Geometry: final body of the model. Coordinates: model frame, mm. A direction names the side the tool comes from. Give positions to 0.01 mm unless a question says otherwise; leave off trailing zeros. Order: outer loops, then holes, each group sorted by start corner. A loop starts at its lowest first (then second) coordinate and runs counter-clockwise, first axis right, second up. Notation, with made-up numbers: (74, -12.5) - (93, -12.5) arc R29 ccw to (93, 7.5) - close; hole circle Ø4 at (78, 21). An arc over 180 degrees is marked (long way). Use one line per item in the form item = value.
from build123d import *

# Parameters (mm, degrees)
F1_DEPTH = 15.24
F2_DEPTH = 12.192
F3_DEPTH = 9.144
F4_DEPTH = 6.096


with BuildPart() as f1:
    # F0 (on Top) → F1 (new body)
    with BuildSketch(Plane.XY):
        Polygon((-19.076721, 37.150636), (-54.891605, 37.150636), (-76.409116, -37.150636), (-40.594233, -37.150636), align=None)
        Polygon((-61.239227, -25.750598), (-46.324576, 25.750598), (-34.24661, 25.750598), (-49.161262, -25.750598), align=None, mode=Mode.SUBTRACT)
    extrude(amount=F1_DEPTH)

    # F0 (on Top) → F2 (join)
    with BuildSketch(Plane.XY):
        Polygon((-6.884721, 37.150636), (-19.076721, 37.150636), (-40.594233, -37.150636), (-24.240132, -37.150636), (-17.038353, -28.016673), (-14.754863, -37.150636), (-5.972206, -37.150636), (15.545306, 37.150636), (5.307279, 37.150636), (-9.230042, -13.047613), (-12.835056, -3.14023), (-21.369147, -12.864963), align=None)
    extrude(amount=F2_DEPTH)

    # F0 (on Top) → F3 (join)
    with BuildSketch(Plane.XY):
        Polygon((43.298501, 37.150636), (15.545306, 37.150636), (-5.972206, -37.150636), (21.78099, -37.150636), (25.299825, -24.999883), (11.423228, -24.999883), (17.365993, -4.479155), (26.523624, -4.479155), (29.117934, 4.479155), (26.523624, 4.479155), (19.960303, 4.479155), (25.932101, 25.100136), (39.808699, 25.100136), align=None)
    extrude(amount=F3_DEPTH)

    # F0 (on Top) → F4 (join)
    with BuildSketch(Plane.XY):
        Polygon((57.90846, 37.150636), (43.298501, 37.150636), (39.808699, 25.100136), (25.299825, -24.999883), (21.78099, -37.150636), (35.253152, -37.150636), (46.813049, 2.766387), (46.813049, -7.282906), (46.813049, -37.150636), (49.582697, -37.150636), (63.912243, -37.150636), (85.429754, 37.150636), (73.237754, 37.150636), (57.90846, -15.782347), align=None)
    extrude(amount=F4_DEPTH)


solid = f1.part
(1) Cut plane B-B on z = 2.5. Give the number of separate pieces and of enclosed holes in the cut face, plus the area to 3 significant figures.
Computed values:
separate_pieces = 1
enclosed_holes = 2
area = 7,960 mm²
(2) Contact query for flat-ended pins moving along their axis: pin 1 Ø5 at (y, z) = (-10, 3) entering from +X; pin 2 Ø5 at (y, z) = (-11, 3) entering from -X; pin 3 Ø4 at (y, z) = (27.5, 2) entering from +X. Output: stop coordinate, or through.
Computed values:
pin_1 = 72.5
pin_2 = -69.56
pin_3 = 83.21
(3) Reachability of faces 4 (the face through (79, 37.151, 3)), 5 (the face through (65.68, 11.05, 3.01)), 6 (the face through (14.353, -14.883, 4.508)), 7 (the face through (-20.69, -32.65, 6.01)), 8 (the face through (18, 1, 9.144)) from +Z, -Z, +X, -X, +Y, -Y: full face, straight path, thin tool, end or side. Return the list, or none.
Computed values:
face_4 = +Z, -Z, +X, -X, +Y
face_5 = +Z, -Z, +Y
face_6 = +Z, -Z
face_7 = +Z, -Z, -Y
face_8 = +Z, +X, -Y
(4) Ray query, line 1 along X through (y, z) = (-20.5, 5.25); line 2 along X through (y, z) = (-12, 11.5); line 3 along X through (y, z) = (14, 9). Return the intervals inside material, ascending.
Computed values:
line_1 = -71.59 to -59.72, -47.64 to 12.73, 26.6 to 40.08, 46.81 to 68.73
line_2 = -69.13 to -57.26, -45.18 to -21.12, -20.61 to -9.61, -8.93 to 1.31
line_3 = -61.6 to -49.73, -37.65 to -13.59, -1.4 to 22.72
(5) Cut plane A-A on z = 10.75. Output: boundary loops of the cut face in (x, y), plus the area to 3 significant figures.
Computed values:
outline = (-76.41, -37.15) - (-24.24, -37.15) - (-17.04, -28.02) - (-14.75, -37.15) - (-5.97, -37.15) - (15.55, 37.15) - (5.31, 37.15) - (-9.23, -13.05) - (-12.84, -3.14) - (-21.37, -12.86) - (-6.88, 37.15) - (-54.89, 37.15) - close; hole (-61.24, -25.75) - (-49.16, -25.75) - (-34.25, 25.75) - (-46.32, 25.75) - close
area = 4,020 mm²
(6) Pull-direction query (X, two-part tool) for faces 1 (the face through (18, -25, 5)), 2 (the face through (3, 1, 0)), 3 (the face through (-29.986, -0.52, 13.695)); classes: released by +X, released by -X, zero draft, split by the parting line, or undercut.
Computed values:
face_1 = undercut
face_2 = zero draft
face_3 = released by +X
(7) Cut plane D-D on y = -32. Output: boundary loops of the cut face in (x, z).
Computed values:
outline = (-74.92, 0) - (-20.18, 0) - (-20.18, 12.19) - (-39.1, 12.19) - (-39.1, 15.24) - (-74.92, 15.24) - close; (-16.04, 0) - (36.74, 0) - (36.74, 6.1) - (23.27, 6.1) - (23.27, 9.14) - (-4.48, 9.14) - (-4.48, 12.19) - (-16.04, 12.19) - close; (46.81, 0) - (65.4, 0) - (65.4, 6.1) - (46.81, 6.1) - close
